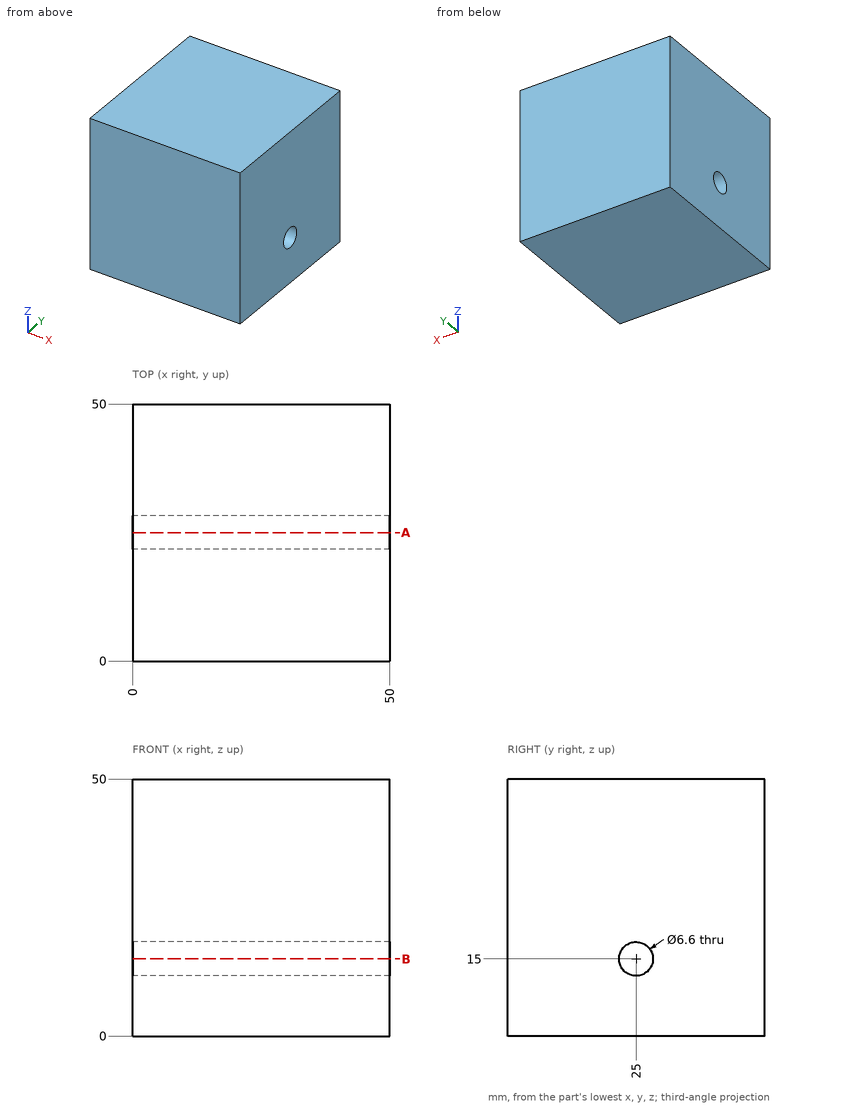
Geometry check sheet. Reference: drawing and pictorial views, mm from the part's lowest x, y, z. Round coordinates to 2 decimals unless told otherwise and drop trailing zeros. Order: outer loops, then holes, each group sorted by start corner. A loop starts at its lowest first (then second) coordinate and runs counter-clockwise, first axis right, second up. Notation, with made-up numbers: M 0.25,-22 L 59.25,-22 A9 ccw 59.25,-16 Z; hole C 6,31 d8. An arc over 180 degrees is marked long. Answer in a Markdown table with one row per item.
(1) Sectioned sample at A-A, the plane y = 25. Record the cut outline in (x, z), and give its area (3 significant figures).
Responses:
| item | result |
|---|---|
| outline | M 0,0 L 50,0 L 50,11.7 L 0,11.7 Z; M 0,18.3 L 50,18.3 L 50,50 L 0,50 Z |
| area | 2,170 mm² |
(2) Sectioned sample at B-B, the plane z = 15. Record the cut outline in (x, y).
Responses:
| item | result |
|---|---|
| outline | M 0,0 L 50,0 L 50,21.7 L 0,21.7 Z; M 0,28.3 L 50,28.3 L 50,50 L 0,50 Z |
(3) Scan lines: probe 1 along Z at (x, y) = (15, 25); probe 2 along Y at (x, z) = (10.5, 12); probe 3 along Y at (x, z) = (30, 13). Record each from-to range of solid material in increasing order. Write a range as from..to.
Responses:
| item | result |
|---|---|
| probe 1 | z = 0..11.7, 18.3..50 |
| probe 2 | y = 0..23.63, 26.37..50 |
| probe 3 | y = 0..22.38, 27.62..50 |
(4) Go/stop test with a flat-tipped pin: P1, Ø3, axis at y = 19, z = 21.5, coming from the -X side. Record where the tip stops, or that it passes through.
Responses:
| item | result |
|---|---|
| P1 | stops at x = 0 |
